For this review, take the finished solid that the model builds, in its own axes (mm). A direction names the side the tool comes from. Coordinates: 2 decimals unless noted, no trailing zeros. Order: outer loops, then holes, each group sorted by start corner. A loop starts at its lowest first (then second) coordinate and runs counter-clockwise, first axis right, second up. Notation, with made-up numbers: M 53,18 L 80,18 A25 ccw 80,30 Z; hole C -3,6 d5. An arc over 180 degrees is marked long. Use one line per item in the form item = value. Start each with the question number.
```python
from build123d import *

# Parameters (mm, degrees)
SKETCH1_W           = 43
SKETCH1_H           = 43
SKETCH1_R           = 1.5
SKETCH1_R_2         = 10
BOSS_EXTRUDE1_DEPTH = 3
CUT_EXTRUDE1_DEPTH  = 3


with BuildPart() as part:
    # Sketch1 → Boss-Extrude1 (new body)
    with BuildSketch(Plane.XY):
        Rectangle(SKETCH1_W, SKETCH1_H)
        with Locations((-12.374368671, 12.374368671)):
            Circle(SKETCH1_R, mode=Mode.SUBTRACT)
        with Locations((12.374368671, -12.374368671)):
            Circle(SKETCH1_R, mode=Mode.SUBTRACT)
        with Locations((12.374368671, 12.374368671)):
            Circle(SKETCH1_R, mode=Mode.SUBTRACT)
        with Locations((-12.374368671, -12.374368671)):
            Circle(SKETCH1_R, mode=Mode.SUBTRACT)
        Circle(SKETCH1_R_2, mode=Mode.SUBTRACT)
    extrude(amount=BOSS_EXTRUDE1_DEPTH)

    # Sketch2 → Cut-Extrude1 (cut)
    with BuildSketch(Plane.XY.offset(3)):
        Polygon((-21.5, -21.5), (21.5, -21.5), (21.5, -18.5), (21.5, -6.5), (18.5, -6.5), (18.5, -18.5), (-18.5, -18.5), (-18.5, -6.5), (-21.5, -6.5), (-21.5, -18.5), align=None)
        Polygon((-21.5, 9.5), (-18.5, 9.5), (-18.5, 18.5), (-9.5, 18.5), (-9.5, 21.5), (-21.5, 21.5), align=None)
        Polygon((21.5, 9.5), (21.5, 21.5), (9.5, 21.5), (9.5, 18.5), (18.5, 18.5), (18.5, 9.5), align=None)
    extrude(amount=-CUT_EXTRUDE1_DEPTH, mode=Mode.SUBTRACT)


solid = part.part
```
1. Consider section B-B, the plane x = 0. Write out the cut boundary in (y, z), plus the area to 3 significant figures.
2. For pin 1 Ø1.5 at (y, z) = (17, 0.5) entering from -X; pin 2 Ø16 at (x, y) = (0, 0) entering from +Z; pin 3 Ø0.9 at (y, z) = (20.5, 1.5) entering from -X; pin 4 Ø1.5 at (x, z) = (19.5, 2) entering from -Y, all flat-tipped, find the tip position at first contact; note any pin that passes through.
3. The part is to be moulded in two halves that separate along X. For faces 1 (the cylindrical face through (-12.7, 10.91, 1.48)), 2 (the flat face through (21.5, 1, 1)), 3 (the flat face through (-20, 9.5, 2)), 4 (the cylindrical face through (-11.57, -11.11, 1.48)), say which applies: pulls with the +X half, pulls with the -X half, needs draft (parallel to the pull), parting line crosses it, or undercut.
4. Consider section A-A, the plane y = 0. Write out the cut boundary in (x, z).
5. Consider section C-C, the plane x = -12. Write out the cut boundary in (y, z).
6. To check wall thickness, follow line 1 (Y direction, x = 0, z = 0.8); line 2 (Y direction, x = 13, z = 0.6); line 3 (X direction, y = -14, z = 1.35). State the ranges of each line that lie inside material, in increasing order.
7. Consider section D-D, the plane z = 1.4. Write out the cut boundary in (x, y), plus the area to 3 significant figures.
8. Tool access review of faces 5 (the flat face through (-18.5, -13, 2)), 6 (the flat face through (-14, 18.5, 2)), 7 (the flat face through (9.5, 20, 2)), 8 (the flat face through (18.5, -12, 2)): name each direction out of +Z, -Z, +X, -X, +Y, -Y from which nothing blocks a thin tool from reaching the whole face with its end or side.
Answers follow:
q1.outline = M -18.5,0 L -10,0 L -10,3 L -18.5,3 Z; M 10,0 L 21.5,0 L 21.5,3 L 10,3 Z
q1.area = 60.0 mm²
q2.pin_1 = -18.5
q2.pin_2 = through
q2.pin_3 = -9.5
q2.pin_4 = -6.5
q3.face_1 = undercut
q3.face_2 = pulls with the +X half
q3.face_3 = needs draft
q3.face_4 = undercut
q4.outline = M -21.5,0 L -10,0 L -10,3 L -21.5,3 Z; M 10,0 L 21.5,0 L 21.5,3 L 10,3 Z
q5.outline = M -18.5,0 L -13.83,0 L -13.83,3 L -18.5,3 Z; M -10.92,0 L 10.92,0 L 10.92,3 L -10.92,3 Z; M 13.83,0 L 18.5,0 L 18.5,3 L 13.83,3 Z
q6.line_1 = -18.5 to -10, 10 to 21.5
q6.line_2 = -18.5 to -13.74, -11.01 to 11.01, 13.74 to 18.5
q6.line_3 = -18.5 to 18.5
q7.outline = M -21.5,-6.5 L -18.5,-6.5 L -18.5,-18.5 L 18.5,-18.5 L 18.5,-6.5 L 21.5,-6.5 L 21.5,9.5 L 18.5,9.5 L 18.5,18.5 L 9.5,18.5 L 9.5,21.5 L -9.5,21.5 L -9.5,18.5 L -18.5,18.5 L -18.5,9.5 L -21.5,9.5 Z; hole C -12.37,-12.37 d3; hole C -12.37,12.37 d3; hole C 0,0 d20; hole C 12.37,-12.37 d3; hole C 12.37,12.37 d3
q7.area = 1,180 mm²
q8.face_5 = +Z, -Z, -X, -Y
q8.face_6 = +Z, -Z, -X, +Y
q8.face_7 = +Z, -Z, +X, +Y
q8.face_8 = +Z, -Z, +X, -Y
